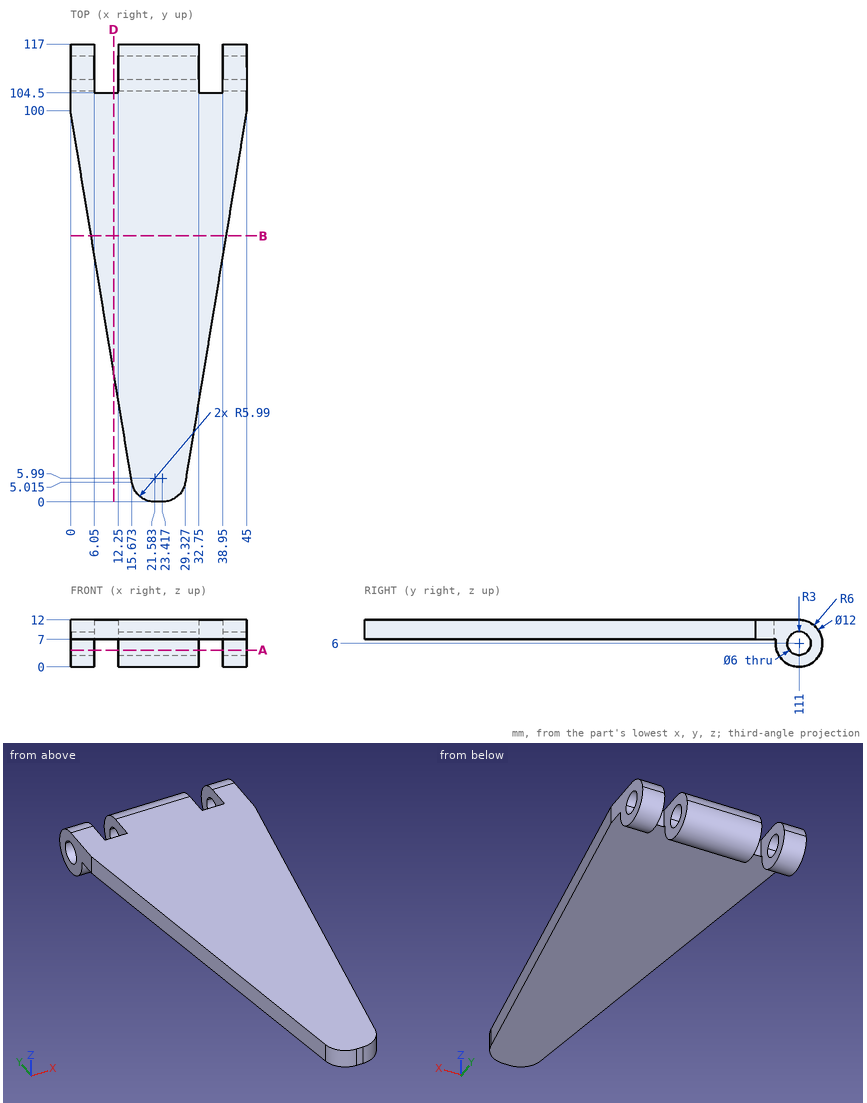
Print and shaded views of the part. All mm, measured from the part's lowest x, y and z. Give positions to 0.01 mm unless a question says otherwise; leave off trailing zeros. Loops run counter-clockwise (first coordinate to the right, second up) from the corner with the lowest first, then second, coordinate; pieces in that order, holes last. Notation, with made-up numbers: (16, 72) -> (57, 72) arc R19 ccw to (57, 94) -> close; hole circle Ø5 at (20.25, 85.25). An arc over 180 degrees is marked (long way). One line per question, with ' | ' between items. Start each with the question number.
1) Cut at A-A (z = 4.25). Give the cut face in (x, y), plus the area to 3 significant figures.
2) Probe L1, parallel to Y at x = 16.5, z = 6; L2, parallel to Z at x = 17.5, y = 111; L3, parallel to Y at x = 3, z = 5 (1 decimal). List the from-to ranges inside material, lowest first.
3) Cut at B-B (y = 68). Give the cut face in (x, z), plus the area to 3 significant figures.
4) Cut at D-D (x = 11). Give the cut face in (y, z).
5) Pin check, flat tips, straight feed: pin 1 (5.5 mm diameter, centred on y = 111, z = 6, fed in from +X); pin 2 (13.5 mm diameter, centred on x = 28.5, y = 48.5, fed in from -Z); pin 3 (2.5 mm diameter, centred on x = 35, z = 9.5, fed in from +Y); pin 4 (1.5 mm diameter, centred on y = 60, z = 7.5, fed in from +X). Stop position of each tip, or through.
Return value:
1) outline: (0, 105.26) -> (6.05, 105.26) -> (6.05, 108.56) -> (0, 108.56) -> close; (0, 113.44) -> (6.05, 113.44) -> (6.05, 116.74) -> (0, 116.74) -> close; (12.25, 105.26) -> (32.75, 105.26) -> (32.75, 108.56) -> (12.25, 108.56) -> close; (12.25, 113.44) -> (32.75, 113.44) -> (32.75, 116.74) -> (12.25, 116.74) -> close; (38.95, 105.26) -> (45, 105.26) -> (45, 108.56) -> (38.95, 108.56) -> close; (38.95, 113.44) -> (45, 113.44) -> (45, 116.74) -> (38.95, 116.74) -> close | area: 215 mm^2
2) L1: 105 to 108, 114 to 117 | L2: 0 to 3, 9 to 12 | L3: 105.1 to 108.2, 113.8 to 116.9
3) outline: (5.28, 7) -> (39.72, 7) -> (39.72, 12) -> (5.28, 12) -> close | area: 172 mm^2
4) outline: (33.33, 7) -> (104.5, 7) -> (104.5, 12) -> (33.33, 12) -> close
5) pin 1: through | pin 2: z = 7 | pin 3: y = 104.5 | pin 4: x = 38.52
